Design review of the part built by this model. Coordinates are the model's own, in mm. A direction names the side the tool comes from. Coordinates: 2 decimals unless noted, no trailing zeros. Write each loop counter-clockwise with the first axis right and the second up, starting at its lowest first coordinate (ties: lowest second). Pieces come first, ordered by that corner, then holes. Notation, with made-up numbers: M -19,73 L -3,73 A9 ccw -3,79 Z; hole C 80,34 d10. An arc over 180 degrees is marked long. Write item = value, one per line.
```python
from build123d import *

# Parameters (mm, degrees)
SKETCH_1_W          = 70
SKETCH_1_H          = 126
EXTRUDE_1_DEPTH     = 2
FILLET_1_R          = 5
SKETCH_2_R          = 2.1
SKETCH_2_R_2        = 1.35
CUT_EXTRUDE_1_DEPTH = 3
SKETCH_3_W          = 45
SKETCH_3_H          = 63
CUT_EXTRUDE_2_DEPTH = 10
FILLET_2_R          = 5


with BuildPart() as part:
    # 草图1 → 凸台-拉伸1 (new body)
    with BuildSketch(Plane.XY):
        Rectangle(SKETCH_1_W, SKETCH_1_H)
    extrude(amount=EXTRUDE_1_DEPTH)

    # 圆角1
    fillet_1_edges = [part.edges().sort_by_distance(p)[0] for p in [
        (35, -63, 1),
        (-35, -63, 1),
        (-35, 63, 1),
        (35, 63, 1),
    ]]
    fillet(fillet_1_edges, radius=FILLET_1_R)

    # 草图2 → 切除-拉伸1 (cut, through all)
    with BuildSketch(Plane.XY.offset(2)):
        with Locations((-25, -58)):
            Circle(SKETCH_2_R)
        with Locations((25, -58)):
            Circle(SKETCH_2_R)
        with Locations((-25, -3)):
            Circle(SKETCH_2_R_2)
        with Locations((-25, 41)):
            Circle(SKETCH_2_R_2)
        with Locations((31, 52.75)):
            Circle(SKETCH_2_R_2)
        with Locations((31, -14.75)):
            Circle(SKETCH_2_R_2)
    extrude(amount=-CUT_EXTRUDE_1_DEPTH, mode=Mode.SUBTRACT)

    # 草图3 → 切除-拉伸2 (cut)
    with BuildSketch(Plane.XY.offset(2)):
        with Locations((2.5, 23.5)):
            Rectangle(SKETCH_3_W, SKETCH_3_H)
    extrude(amount=-CUT_EXTRUDE_2_DEPTH, mode=Mode.SUBTRACT)

    # 圆角2
    fillet_2_edges = [part.edges().sort_by_distance(p)[0] for p in [
        (25, 55, 1),
        (25, -8, 1),
        (-20, -8, 1),
        (-20, 55, 1),
    ]]
    fillet(fillet_2_edges, radius=FILLET_2_R)


solid = part.part
```
Q1. Consider section B-B, the plane y = 41. State the section outline as (x, z) points.
Check result:
outline = M -35,0 L -26.35,0 L -26.35,2 L -35,2 Z; M -23.65,0 L -20,0 L -20,2 L -23.65,2 Z; M 25,0 L 35,0 L 35,2 L 25,2 Z
Q2. Machinability: for faces 5 (the cylindrical face through (-18, -7, 1)), 6 (the cylindrical face through (-34, -61, 1)), which of the approach directions +Z, -Z, +X, -X, +Y, -Y give a long, thin tool a straight path to every point of the face, cutting with its end or side? Answer none if there is none.
Check result:
face_5 = +Z, -Z
face_6 = +Z, -Z, -X, -Y
Q3. Consider section C-C, the plane x = 8. State the section outline as (y, z) points.
Check result:
outline = M -63,0 L -8,0 L -8,2 L -63,2 Z; M 55,0 L 63,0 L 63,2 L 55,2 Z
Q4. Wall thickness on line 1 (Y direction, x = -25, z = 0.5); line 2 (X direction, y = 21.5, z = 1.25); line 3 (Y direction, x = 0, z = 1.7): over which ranges is each line inside the solid? List them lowest first.
Check result:
line_1 = -63 to -60.1, -55.9 to -4.35, -1.65 to 39.65, 42.35 to 63
line_2 = -35 to -20, 25 to 35
line_3 = -63 to -8, 55 to 63
Q5. Consider section A-A, the plane x = -25. State the section outline as (y, z) points.
Check result:
outline = M -63,0 L -60.1,0 L -60.1,2 L -63,2 Z; M -55.9,0 L -4.35,0 L -4.35,2 L -55.9,2 Z; M -1.65,0 L 39.65,0 L 39.65,2 L -1.65,2 Z; M 42.35,0 L 63,0 L 63,2 L 42.35,2 Z
Q6. The part is to be moulded in two halves that separate along Y. For faces 1 (the flat face through (0, -13, 0)), 2 (the cylindrical face through (23, -7, 1)), 3 (the cylindrical face through (-24.38, 39.8, 1.01)), 4 (the cylindrical face through (-34, 61, 1)), say which applies: +Y half, -Y half, draft (parallel to the pull), parting line (faces both ways), or undercut.
Check result:
face_1 = draft
face_2 = undercut
face_3 = undercut
face_4 = +Y half
Q7. Consider section D-D, the plane y = 19.5. State the section outline as (x, z) points, and give its area (3 significant figures).
Check result:
outline = M -35,0 L -20,0 L -20,2 L -35,2 Z; M 25,0 L 35,0 L 35,2 L 25,2 Z
area = 50.0 mm²
